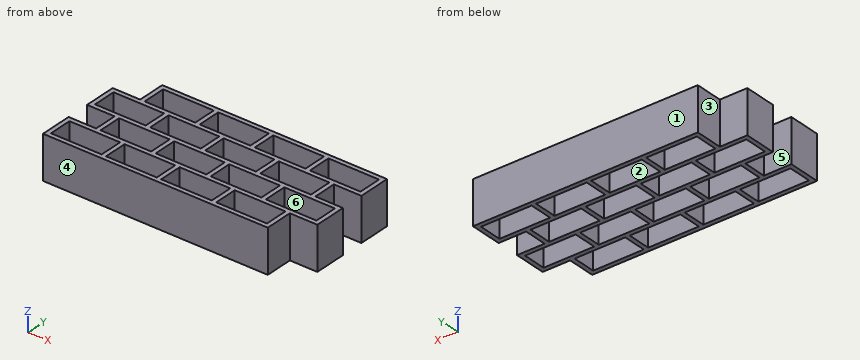
```python
from build123d import *

# Parameters (mm, degrees)
EXTRUDE_1_DEPTH = 4


with BuildPart() as part:
    # 草图1 → 凸台-拉伸1 (new body)
    with BuildSketch(Plane.XY):
        Polygon((-2.75, 1.48), (-2.75, -1.48), (2.34, -1.48), (2.75, -1.48), (7.43, -1.48), (7.84, -1.48), (12.52, -1.48), (12.93, -1.48), (18.02, -1.48), (18.02, 1.07), (20.565, 1.07), (20.565, 4.03), (18.02, 4.03), (18.02, 6.17), (20.565, 6.17), (20.565, 9.13), (15.475, 9.13), (15.065, 9.13), (10.385, 9.13), (9.975, 9.13), (5.295, 9.13), (4.885, 9.13), (-0.205, 9.13), (-0.205, 6.58), (-2.75, 6.58), (-2.75, 3.62), (-0.205, 3.62), (-0.205, 1.48), align=None)
        Polygon((-2.34, 1.07), (-0.205, 1.07), (0.205, 1.07), (2.34, 1.07), (2.34, 0.205), (2.34, -0.205), (2.34, -1.07), (0.205, -1.07), (-0.205, -1.07), (-2.34, -1.07), (-2.34, -0.205), (-2.34, 0.205), align=None, mode=Mode.SUBTRACT)
        Polygon((2.75, 0.205), (2.75, 1.07), (4.885, 1.07), (5.295, 1.07), (7.43, 1.07), (7.43, 0.205), (7.43, -0.205), (7.43, -1.07), (5.295, -1.07), (4.885, -1.07), (2.75, -1.07), (2.75, -0.205), align=None, mode=Mode.SUBTRACT)
        Polygon((4.885, 1.48), (2.75, 1.48), (2.34, 1.48), (0.205, 1.48), (0.205, 2.345), (0.205, 2.755), (0.205, 3.62), (2.34, 3.62), (2.75, 3.62), (4.885, 3.62), (4.885, 2.755), (4.885, 2.345), align=None, mode=Mode.SUBTRACT)
        Polygon((9.975, 1.48), (7.84, 1.48), (7.43, 1.48), (5.295, 1.48), (5.295, 2.345), (5.295, 2.755), (5.295, 3.62), (7.43, 3.62), (7.84, 3.62), (9.975, 3.62), (9.975, 2.755), (9.975, 2.345), align=None, mode=Mode.SUBTRACT)
        Polygon((7.84, 0.205), (7.84, 1.07), (9.975, 1.07), (10.385, 1.07), (12.52, 1.07), (12.52, 0.205), (12.52, -0.205), (12.52, -1.07), (10.385, -1.07), (9.975, -1.07), (7.84, -1.07), (7.84, -0.205), align=None, mode=Mode.SUBTRACT)
        Polygon((12.93, 0.205), (12.93, 1.07), (15.065, 1.07), (15.475, 1.07), (17.61, 1.07), (17.61, 0.205), (17.61, -0.205), (17.61, -1.07), (15.475, -1.07), (15.065, -1.07), (12.93, -1.07), (12.93, -0.205), align=None, mode=Mode.SUBTRACT)
        Polygon((15.065, 1.48), (12.93, 1.48), (12.52, 1.48), (10.385, 1.48), (10.385, 2.345), (10.385, 2.755), (10.385, 3.62), (12.52, 3.62), (12.93, 3.62), (15.065, 3.62), (15.065, 2.755), (15.065, 2.345), align=None, mode=Mode.SUBTRACT)
        Polygon((20.155, 3.62), (20.155, 2.755), (20.155, 2.345), (20.155, 1.48), (18.02, 1.48), (17.61, 1.48), (15.475, 1.48), (15.475, 2.345), (15.475, 2.755), (15.475, 3.62), (17.61, 3.62), (18.02, 3.62), align=None, mode=Mode.SUBTRACT)
        Polygon((-0.205, 4.03), (-2.34, 4.03), (-2.34, 4.895), (-2.34, 5.305), (-2.34, 6.17), (-0.205, 6.17), (0.205, 6.17), (2.34, 6.17), (2.34, 5.305), (2.34, 4.895), (2.34, 4.03), (0.205, 4.03), align=None, mode=Mode.SUBTRACT)
        Polygon((4.885, 4.03), (2.75, 4.03), (2.75, 4.895), (2.75, 5.305), (2.75, 6.17), (4.885, 6.17), (5.295, 6.17), (7.43, 6.17), (7.43, 5.305), (7.43, 4.895), (7.43, 4.03), (5.295, 4.03), align=None, mode=Mode.SUBTRACT)
        Polygon((4.885, 6.58), (2.75, 6.58), (2.34, 6.58), (0.205, 6.58), (0.205, 7.445), (0.205, 7.855), (0.205, 8.72), (2.34, 8.72), (2.75, 8.72), (4.885, 8.72), (4.885, 7.855), (4.885, 7.445), align=None, mode=Mode.SUBTRACT)
        Polygon((5.295, 7.445), (5.295, 7.855), (5.295, 8.72), (7.43, 8.72), (7.84, 8.72), (9.975, 8.72), (9.975, 7.855), (9.975, 7.445), (9.975, 6.58), (7.84, 6.58), (7.43, 6.58), (5.295, 6.58), align=None, mode=Mode.SUBTRACT)
        Polygon((9.975, 4.03), (7.84, 4.03), (7.84, 4.895), (7.84, 5.305), (7.84, 6.17), (9.975, 6.17), (10.385, 6.17), (12.52, 6.17), (12.52, 5.305), (12.52, 4.895), (12.52, 4.03), (10.385, 4.03), align=None, mode=Mode.SUBTRACT)
        Polygon((15.065, 4.03), (12.93, 4.03), (12.93, 4.895), (12.93, 5.305), (12.93, 6.17), (15.065, 6.17), (15.475, 6.17), (17.61, 6.17), (17.61, 5.305), (17.61, 4.895), (17.61, 4.03), (15.475, 4.03), align=None, mode=Mode.SUBTRACT)
        Polygon((10.385, 7.445), (10.385, 7.855), (10.385, 8.72), (12.52, 8.72), (12.93, 8.72), (15.065, 8.72), (15.065, 7.855), (15.065, 7.445), (15.065, 6.58), (12.93, 6.58), (12.52, 6.58), (10.385, 6.58), align=None, mode=Mode.SUBTRACT)
        Polygon((15.475, 7.445), (15.475, 7.855), (15.475, 8.72), (17.61, 8.72), (18.02, 8.72), (20.155, 8.72), (20.155, 6.58), (18.02, 6.58), (17.61, 6.58), (15.475, 6.58), align=None, mode=Mode.SUBTRACT)
    extrude(amount=EXTRUDE_1_DEPTH)


solid = part.part
```
Geometry: final body of the model. Coordinates: model frame, mm. Face numbers are marked on the shaded views. A direction names the side the tool comes from. Coordinates: 2 decimals unless noted, no trailing zeros. Order: outer loops, then holes, each group sorted by start corner. A loop starts at its lowest first (then second) coordinate and runs counter-clockwise, first axis right, second up. Notation, with made-up numbers: (-18.5, -2.75) - (22.5, -2.75) arc R11 cw to (22.5, 16.25) - close; hole circle Ø9 at (53.25, 0.5). An arc over 180 degrees is marked (long way). Return JSON: item names as keys, results as strings. Group by question number.
1. Pin query (flat end, axial travel): pin 1 (2 mm diameter, centred on x = -2, z = 3, fed in from +Y); pin 2 (1.7 mm diameter, centred on y = 0, z = 1.5, fed in from +X); pin 3 (1.3 mm diameter, centred on x = 19.5, z = 1, fed in from -Y); pin 4 (2 mm diameter, centred on x = 9, y = 0, fed in from -Z). Return the tip coordinate at first contact, or that it passes through.
2. Set-up query: the marked faces 4, 5 and 6. Return all of +Z, -Z, +X, -X, +Y, -Y with unobstructed straight access to the full face (end or side cutting, diameter ignored); none if empty.
3. Cut plane D-D (z = 0.3). Count the separate pieces of the cut face and the enclosed holes in it, plus the area to 3 significant figures.
4. Cut plane A-A (x = 18.25). Output: boundary loops of the cut face in (y, z).
5. Material intervals for line 1 along X through (y, z) = (3, 0.3) (3 decimals); line 2 along Y through (x, z) = (19.75, 1.9); line 3 along Y through (x, z) = (-0.5, 0.7), sorted ascending. Write a range as [from, to].
6. Pull-direction query (X, two-part tool) for the marked faces 1, 2 and 3; classes: pulls with the +X half, pulls with the -X half, needs draft (parallel to the pull), parting line crosses it, or undercut.
7. Cut plane B-B (y = 2.5). Output: boundary loops of the cut face in (x, z) (3 decimals), plus the area to 3 significant figures.
8. Cut plane C-C (x = 7). Output: boundary loops of the cut face in (y, z), plus the area to 3 significant figures.
Resolved:
{
 "1": {"pin 1": "stops at y = 6.58", "pin 2": "stops at x = 18.02", "pin 3": "stops at y = 1.07", "pin 4": "passes through"},
 "2": {"face 4": "+Z, -Z, +X, -X, -Y", "face 5": "+Z, -Z, -X", "face 6": "+Z, -Z"},
 "3": {"separate pieces": "1", "enclosed holes": "16", "area": "63.3 mm²"},
 "4": {"outline": "(1.07, 0) - (1.48, 0) - (1.48, 4) - (1.07, 4) - close; (3.62, 0) - (4.03, 0) - (4.03, 4) - (3.62, 4) - close; (6.17, 0) - (6.58, 0) - (6.58, 4) - (6.17, 4) - close; (8.72, 0) - (9.13, 0) - (9.13, 4) - (8.72, 4) - close"},
 "5": {"line 1": "x = [-0.205, 0.205], [4.885, 5.295], [9.975, 10.385], [15.065, 15.475], [20.155, 20.565]", "line 2": "y = [1.07, 1.48], [3.62, 4.03], [6.17, 6.58], [8.72, 9.13]", "line 3": "y = [-1.48, -1.07], [1.07, 1.48], [3.62, 4.03], [6.17, 6.58]"},
 "6": {"face 1": "needs draft", "face 2": "undercut", "face 3": "pulls with the -X half"},
 "7": {"outline": "(-0.205, 0) - (0.205, 0) - (0.205, 4) - (-0.205, 4) - close; (4.885, 0) - (5.295, 0) - (5.295, 4) - (4.885, 4) - close; (9.975, 0) - (10.385, 0) - (10.385, 4) - (9.975, 4) - close; (15.065, 0) - (15.475, 0) - (15.475, 4) - (15.065, 4) - close; (20.155, 0) - (20.565, 0) - (20.565, 4) - (20.155, 4) - close", "area": "8.20 mm²"},
 "8": {"outline": "(-1.48, 0) - (-1.07, 0) - (-1.07, 4) - (-1.48, 4) - close; (1.07, 0) - (1.48, 0) - (1.48, 4) - (1.07, 4) - close; (3.62, 0) - (4.03, 0) - (4.03, 4) - (3.62, 4) - close; (6.17, 0) - (6.58, 0) - (6.58, 4) - (6.17, 4) - close; (8.72, 0) - (9.13, 0) - (9.13, 4) - (8.72, 4) - close", "area": "8.20 mm²"}
}
